Answer from the drawing. Dimensions are ordinates in mm from the lowest x, y and z of the part. A direction names the side the tool comes from. Round coordinates to 2 decimals unless told otherwise and drop trailing zeros. Write each loop counter-clockwise with the first axis right and the second up, starting at its lowest first coordinate (ties: lowest second). Pieces come first, ordered by that corner, then holes. Notation, with made-up numbers: (39.25, -26.75) - (87.25, -26.75) arc R12 ccw to (87.25, -15.75) - close; hole circle Ø10 at (35.25, -3.5). An arc over 180 degrees is marked (long way). Use a Markdown table: item, result. Add a question column.
1) A cutting plane is placed at A-A (y = 4). Give the vertices of the cut face in (x, z).
2) A cutting plane is placed at C-C (x = 8). Give the vertices of the cut face in (y, z), then the cut area to 3 significant figures.
3) A tool of negligible diameter and unlimited length cuts with its end or side. For the marked faces 4, 5 and 6, from which of +Z, -Z, +X, -X, +Y, -Y can it reach the whole face along a straight path? Write none if from no direction.
4) Each of these flat-tipped pins is pushed along its axis until it touches: P1, Ø3, axis at y = 5, z = 7, coming from the +X side; P2, Ø5, axis at y = 4, z = 5, coming from the -X side; P3, Ø2.5, axis at x = 16, z = 3.5, coming from the -Y side; P4, Ø1.8, axis at y = 11, z = 5, coming from the +X side. Where does it stop, or does it pass through?
5) Find the intervals of material crossed by probe 1 along Y at (x, z) = (5.75, 5); probe 2 along X at (y, z) = (6.25, 3.25); probe 3 along Y at (x, z) = (2.25, 3.5), in increasing order. Write a range as from..to.
6) A cutting plane is placed at D-D (y = 11.75). Give the vertices of the cut face in (x, z), then the cut area to 3 significant figures.
7) Determine the mould class of the marked faces 1, 2 and 3 for opening direction Z: +Z half, -Z half, draft (parallel to the pull), parting line (faces both ways), or undercut.
8) A cutting plane is placed at B-B (z = 5.75). Give the vertices of the cut face in (x, y), then the cut area to 3 significant figures.
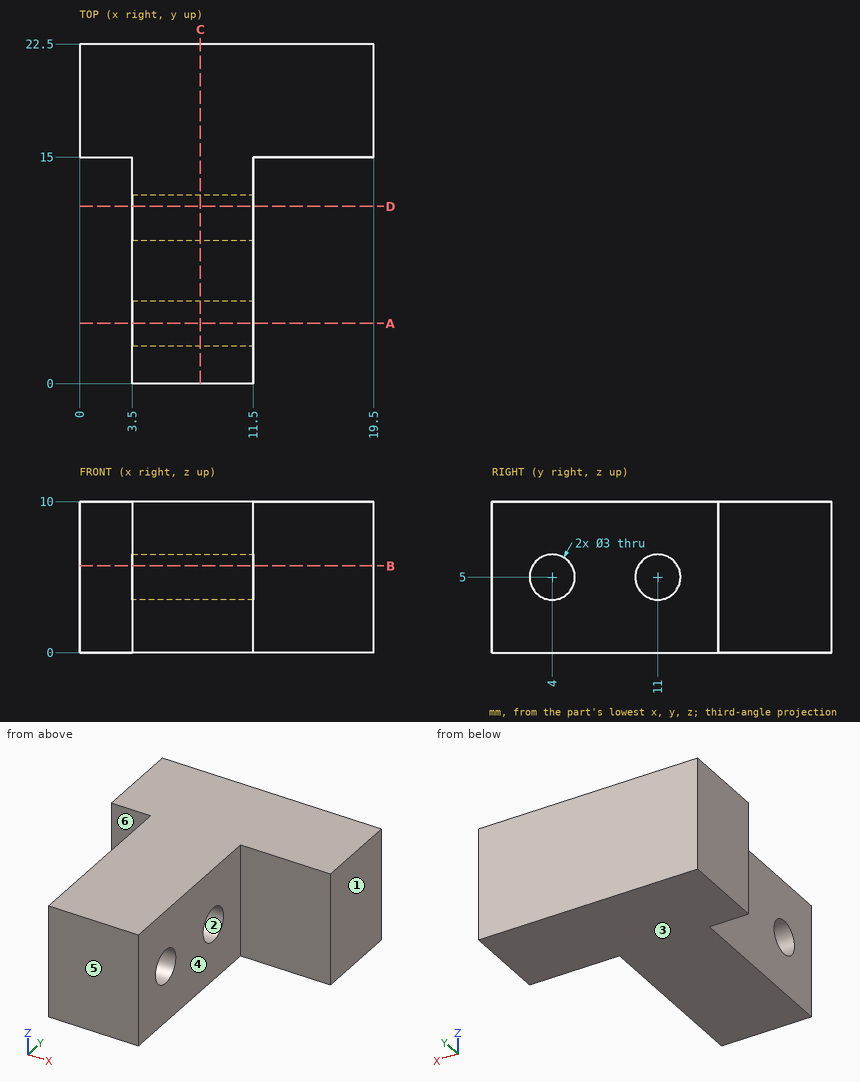
Entries:
| question | item | result |
|---|---|---|
| 1 | outline | (3.5, 0) - (11.5, 0) - (11.5, 3.5) - (3.5, 3.5) - close; (3.5, 6.5) - (11.5, 6.5) - (11.5, 10) - (3.5, 10) - close |
| 2 | outline | (0, 0) - (22.5, 0) - (22.5, 10) - (0, 10) - close; hole circle Ø3 at (4, 5); hole circle Ø3 at (11, 5) |
| 2 | area | 211 mm² |
| 3 | face 4 | +Z, -Z, +X, -Y |
| 3 | face 5 | +Z, -Z, +X, -X, -Y |
| 3 | face 6 | +Z, -Z, -X, -Y |
| 4 | P1 | stops at x = 11.5 |
| 4 | P2 | stops at x = 3.5 |
| 4 | P3 | stops at y = 15 |
| 4 | P4 | passes through |
| 5 | probe 1 | y = 0..2.5, 5.5..9.5, 12.5..22.5 |
| 5 | probe 2 | x = 3.5..11.5 |
| 5 | probe 3 | y = 15..22.5 |
| 6 | outline | (3.5, 0) - (11.5, 0) - (11.5, 3.7) - (3.5, 3.7) - close; (3.5, 6.3) - (11.5, 6.3) - (11.5, 10) - (3.5, 10) - close |
| 6 | area | 59.2 mm² |
| 7 | face 1 | draft |
| 7 | face 2 | undercut |
| 7 | face 3 | -Z half |
| 8 | outline | (0, 15) - (3.5, 15) - (3.5, 12.3) - (11.5, 12.3) - (11.5, 15) - (19.5, 15) - (19.5, 22.5) - (0, 22.5) - close; (3.5, 0) - (11.5, 0) - (11.5, 2.7) - (3.5, 2.7) - close; (3.5, 5.3) - (11.5, 5.3) - (11.5, 9.7) - (3.5, 9.7) - close |
| 8 | area | 225 mm² |
